Could you check a few things on this model? Use its own coordinates, in mm. A direction names the side the tool comes from. Coordinates: 2 decimals unless noted, no trailing zeros. One line per question, with ' | ' between items. Start each with the question number.
from build123d import *
from OCP.BRepFilletAPI import BRepFilletAPI_MakeChamfer

# Parameters (mm, degrees)
SKETCH1_W                       = 16.6
SKETCH1_H                       = 11.5
BOSS_EXTRUDE1_DEPTH             = 10
SKETCH2_W                       = 21
SKETCH2_H                       = 14.8
BOSS_EXTRUDE2_DEPTH             = 1.5
SKETCH3_W                       = 0.5
SKETCH3_H                       = 5
BOSS_EXTRUDE3_DEPTH             = 8
SKETCH4_W                       = 0.5
SKETCH4_H                       = 0.4
CUT_EXTRUDE1_DEPTH              = 22.623424798
BOSS_EXTRUDE4_REACH             = 19.241
SKETCH5_W                       = 0.75
SKETCH5_H                       = 2.5
BOSS_EXTRUDE4_DIRECTION_2_REACH = 19.241
BOSS_EXTRUDE5_DEPTH             = 2.8
BOSS_EXTRUDE5_DEPTH_BACK        = 2.8
CHAMFER1_SIZE                   = 1.8
CHAMFER1_SIZE2                  = 1.039230485
BOSS_EXTRUDE6_DEPTH             = 4.65
SKETCH9_W                       = 1.1
SKETCH9_H                       = 0.45
BOSS_EXTRUDE7_DEPTH             = 1.9
CHAMFER2_SIZE                   = 0.5
CHAMFER2_SIZE2                  = 0.288675135
SCALE2_SCALE                    = 0.7


with BuildPart() as part:
    # Sketch1 → Boss-Extrude1 (new body)
    with BuildSketch(Plane.XY):
        Rectangle(SKETCH1_W, SKETCH1_H)
    extrude(amount=BOSS_EXTRUDE1_DEPTH)

    # Sketch2 → Boss-Extrude2 (add)
    with BuildSketch(Plane.XY.offset(10)):
        Rectangle(SKETCH2_W, SKETCH2_H)
    extrude(amount=BOSS_EXTRUDE2_DEPTH)

    # Sketch3 → Boss-Extrude3 (add)
    with BuildSketch(Plane(origin=(0, 0, 0), x_dir=(-1, 0, 0), z_dir=(0, 0, -1))):
        with Locations((-6, 0)):
            Rectangle(SKETCH3_W, SKETCH3_H)
        Rectangle(SKETCH3_W, SKETCH3_H)
    extrude(amount=BOSS_EXTRUDE3_DEPTH)

    # Sketch4 → Cut-Extrude1 (cut, through all)
    with BuildSketch(Plane(origin=(6.25, 0, 0), x_dir=(0, 0, -1), z_dir=(1, 0, 0))):
        with Locations((2.25, 2.3)):
            Rectangle(SKETCH4_W, SKETCH4_H)
        with BuildLine():
            Line((0, 0.75), (0, -0.75))
            ThreePointArc((0, -0.75), (0.75, 0), (0, 0.75))
        make_face()
        Polygon((6.5, 2.5), (8, 1.449688693), (8, 2.5), align=None)
        with BuildLine():
            Line((5.432692308, 0.612598863), (6.3, 0))
            Line((6.3, 0), (5.432692308, -0.612598863))
            ThreePointArc((5.432692308, -0.612598863), (4.25, 0), (5.432692308, 0.612598863))
        make_face()
        Polygon((8, -2.5), (8, -1.449688693), (6.5, -2.5), align=None)
        with Locations((2.25, -2.3)):
            Rectangle(SKETCH4_W, SKETCH4_H)
    extrude(amount=-CUT_EXTRUDE1_DEPTH, mode=Mode.SUBTRACT)

    # Boss-Extrude4: up to this face of the body (flat: up to its plane)
    boss_extrude4_end = Plane(part.part.faces().sort_by_distance((0, 5.75, 5))[0])
    # Sketch5 → Boss-Extrude4 (add, up to the picked face)
    with BuildSketch(Plane(origin=(0, 0, 0), x_dir=(1, 0, 0), z_dir=(0, 1, 0)), mode=Mode.PRIVATE) as boss_extrude4_sk1:
        with Locations((-8.675, -1.25)):
            Rectangle(SKETCH5_W, SKETCH5_H)
    boss_extrude4_tool1 = split(extrude(boss_extrude4_sk1.sketch, amount=BOSS_EXTRUDE4_REACH, mode=Mode.PRIVATE), bisect_by=boss_extrude4_end, keep=Keep.BOTH, mode=Mode.PRIVATE)
    boss_extrude4 = boss_extrude4_tool1.solids().sort_by(Axis((-8.675, 0, 1.25), (0, 1, 0)))[0]
    add(boss_extrude4)

    # Boss-Extrude4 direction 2: up to this face of the body (flat: up to its plane)
    boss_extrude4_direction_2_end = Plane(part.part.faces().sort_by_distance((0, -5.75, 5))[0])
    # Sketch5 → Boss-Extrude4 direction 2 (add, up to the picked face)
    with BuildSketch(Plane(origin=(0, 0, 0), x_dir=(1, 0, 0), z_dir=(0, 1, 0)), mode=Mode.PRIVATE) as boss_extrude4_direction_2_sk1:
        with Locations((-8.675, -1.25)):
            Rectangle(SKETCH5_W, SKETCH5_H)
    boss_extrude4_direction_2_tool1 = split(extrude(boss_extrude4_direction_2_sk1.sketch, amount=-BOSS_EXTRUDE4_DIRECTION_2_REACH, mode=Mode.PRIVATE), bisect_by=boss_extrude4_direction_2_end, keep=Keep.BOTH, mode=Mode.PRIVATE)
    boss_extrude4_direction_2 = boss_extrude4_direction_2_tool1.solids().sort_by(Axis((-8.675, 0, 1.25), (0, -1, 0)))[0]
    add(boss_extrude4_direction_2)

    # Mirror1: Boss-Extrude4, Boss-Extrude4 direction 2 across plane
    add(boss_extrude4.mirror(Plane(origin=(0, 0, 0), x_dir=(0, 0, 1), z_dir=(1, 0, 0))))
    add(boss_extrude4_direction_2.mirror(Plane(origin=(0, 0, 0), x_dir=(0, 0, 1), z_dir=(1, 0, 0))))

    # Sketch6 → Boss-Extrude5 (add, two sides: drawn at the far end of the back side and taken through both)
    with BuildSketch(Plane(origin=(0, 0, 0), x_dir=(1, 0, 0), z_dir=(0, 1, 0)).offset(-BOSS_EXTRUDE5_DEPTH_BACK)):
        with BuildLine():
            Line((-9.05, -2.5), (-10.124907983, -5.653347952))
            ThreePointArc((-10.124907983, -5.653347952), (-10.231819447, -6.312838644), (-10.115557515, -6.970745323))
            Line((-10.115557515, -6.970745323), (-9.056614332, -9.938626949))
            Line((-9.056614332, -9.938626949), (-9.034716365, -10))
            Line((-9.034716365, -10), (-8.3, -10))
            Line((-8.3, -10), (-8.3, -9.827371619))
            Line((-8.3, -9.827371619), (-8.350231447, -9.686588817))
            Line((-8.350231447, -9.686588817), (-9.438479941, -6.636573707))
            ThreePointArc((-9.438479941, -6.636573707), (-9.496610907, -6.307620368), (-9.443155175, -5.977875022))
            Line((-9.443155175, -5.977875022), (-8.34011069, -2.741985882))
            Line((-8.34011069, -2.741985882), (-8.3, -2.624317241))
            Line((-8.3, -2.624317241), (-8.3, -2.5))
            Line((-8.3, -2.5), (-9.05, -2.5))
        make_face()
        with BuildLine():
            Line((8.3, -9.827371619), (8.350231447, -9.686588817))
            Line((8.350231447, -9.686588817), (9.438479941, -6.636573707))
            ThreePointArc((9.438479941, -6.636573707), (9.496610907, -6.307620368), (9.443155175, -5.977875022))
            Line((9.443155175, -5.977875022), (8.34011069, -2.741985882))
            Line((8.34011069, -2.741985882), (8.3, -2.624317241))
            Line((8.3, -2.624317241), (8.3, -2.5))
            Line((8.3, -2.5), (9.05, -2.5))
            Line((9.05, -2.5), (10.124907983, -5.653347952))
            ThreePointArc((10.124907983, -5.653347952), (10.231819447, -6.312838644), (10.115557515, -6.970745323))
            Line((10.115557515, -6.970745323), (9.056614332, -9.938626949))
            Line((9.056614332, -9.938626949), (9.034716365, -10))
            Line((9.034716365, -10), (8.3, -10))
            Line((8.3, -10), (8.3, -9.827371619))
        make_face()
    extrude(amount=BOSS_EXTRUDE5_DEPTH + BOSS_EXTRUDE5_DEPTH_BACK)

    # Chamfer1
    chamfer1_edges = [part.edges().sort_by_distance(p)[0] for p in [
        (10.5, 0, 11.5),
        (0, 7.4, 11.5),
        (-10.5, 0, 11.5),
        (0, -7.4, 11.5),
    ]]
    chamfer1_side = [part.faces().sort_by_distance(p)[0] for p in [
        (0, 0, 11.5),
    ]]
    chamfer(chamfer1_edges, length=CHAMFER1_SIZE, length2=CHAMFER1_SIZE2, reference=chamfer1_side[0])

    # Sketch7 → Boss-Extrude6 (add, symmetric)
    with BuildSketch(Plane(origin=(0, 0, 0), x_dir=(1, 0, 0), z_dir=(0, 1, 0))):
        with BuildLine():
            Line((-7.2, -11.5), (-3.398718251, -16.8))
            add(Edge.make_bspline(
                [(-3.398718251, -16.8), (0.927387699, -12.334784825), (7.2, -11.5)],
                knots=[0, 0, 0, 1, 1, 1], degree=2))
            Line((7.2, -11.5), (-7.2, -11.5))
        make_face()
    extrude(amount=BOSS_EXTRUDE6_DEPTH, both=True)

    # Sketch9 → Boss-Extrude7 (add)
    with BuildSketch(Plane(origin=(0, 0, 10), x_dir=(-1, 0, 0), z_dir=(0, 0, -1))):
        with Locations((-7.425, 5.975)):
            Rectangle(SKETCH9_W, SKETCH9_H)
        with Locations((-2.475, 5.975)):
            Rectangle(SKETCH9_W, SKETCH9_H)
        with Locations((2.475, 5.975)):
            Rectangle(SKETCH9_W, SKETCH9_H)
        with Locations((7.425, 5.975)):
            Rectangle(SKETCH9_W, SKETCH9_H)
        with Locations((7.425, -5.975)):
            Rectangle(SKETCH9_W, SKETCH9_H)
        with Locations((2.475, -5.975)):
            Rectangle(SKETCH9_W, SKETCH9_H)
        with Locations((-2.475, -5.975)):
            Rectangle(SKETCH9_W, SKETCH9_H)
        with Locations((-7.425, -5.975)):
            Rectangle(SKETCH9_W, SKETCH9_H)
    extrude(amount=BOSS_EXTRUDE7_DEPTH)

    # Chamfer2: one chamfer whose edges measure the first distance from different faces: ONE call of the kernel's chamfer builder (chamfer() names one face for all edges)
    chamfer2_edges_1 = [part.edges().sort_by_distance(p)[0] for p in [
        (7.425, 6.2, 8.1),
    ]]
    chamfer2_side_1 = [part.faces().sort_by_distance(p)[0] for p in [
        (7.425, 6.2, 9.05),
    ]]
    chamfer2_edges_2 = [part.edges().sort_by_distance(p)[0] for p in [
        (2.475, 6.2, 8.1),
    ]]
    chamfer2_side_2 = [part.faces().sort_by_distance(p)[0] for p in [
        (2.475, 6.2, 9.05),
    ]]
    chamfer2_edges_3 = [part.edges().sort_by_distance(p)[0] for p in [
        (-2.475, 6.2, 8.1),
    ]]
    chamfer2_side_3 = [part.faces().sort_by_distance(p)[0] for p in [
        (-2.475, 6.2, 9.05),
    ]]
    chamfer2_edges_4 = [part.edges().sort_by_distance(p)[0] for p in [
        (-7.425, 6.2, 8.1),
    ]]
    chamfer2_side_4 = [part.faces().sort_by_distance(p)[0] for p in [
        (-7.425, 6.2, 9.05),
    ]]
    chamfer2_edges_5 = [part.edges().sort_by_distance(p)[0] for p in [
        (-7.425, -6.2, 8.1),
    ]]
    chamfer2_side_5 = [part.faces().sort_by_distance(p)[0] for p in [
        (-7.425, -6.2, 9.05),
    ]]
    chamfer2_edges_6 = [part.edges().sort_by_distance(p)[0] for p in [
        (-2.475, -6.2, 8.1),
    ]]
    chamfer2_side_6 = [part.faces().sort_by_distance(p)[0] for p in [
        (-2.475, -6.2, 9.05),
    ]]
    chamfer2_edges_7 = [part.edges().sort_by_distance(p)[0] for p in [
        (2.475, -6.2, 8.1),
    ]]
    chamfer2_side_7 = [part.faces().sort_by_distance(p)[0] for p in [
        (2.475, -6.2, 9.05),
    ]]
    chamfer2_edges_8 = [part.edges().sort_by_distance(p)[0] for p in [
        (7.425, -6.2, 8.1),
    ]]
    chamfer2_side_8 = [part.faces().sort_by_distance(p)[0] for p in [
        (7.425, -6.2, 9.05),
    ]]
    chamfer2 = BRepFilletAPI_MakeChamfer(part.part.solid().wrapped)
    for e in chamfer2_edges_1:
        chamfer2.Add(CHAMFER2_SIZE, CHAMFER2_SIZE2, e.wrapped, chamfer2_side_1[0].wrapped)  # the first distance lies on this face
    for e in chamfer2_edges_2:
        chamfer2.Add(CHAMFER2_SIZE, CHAMFER2_SIZE2, e.wrapped, chamfer2_side_2[0].wrapped)  # the first distance lies on this face
    for e in chamfer2_edges_3:
        chamfer2.Add(CHAMFER2_SIZE, CHAMFER2_SIZE2, e.wrapped, chamfer2_side_3[0].wrapped)  # the first distance lies on this face
    for e in chamfer2_edges_4:
        chamfer2.Add(CHAMFER2_SIZE, CHAMFER2_SIZE2, e.wrapped, chamfer2_side_4[0].wrapped)  # the first distance lies on this face
    for e in chamfer2_edges_5:
        chamfer2.Add(CHAMFER2_SIZE, CHAMFER2_SIZE2, e.wrapped, chamfer2_side_5[0].wrapped)  # the first distance lies on this face
    for e in chamfer2_edges_6:
        chamfer2.Add(CHAMFER2_SIZE, CHAMFER2_SIZE2, e.wrapped, chamfer2_side_6[0].wrapped)  # the first distance lies on this face
    for e in chamfer2_edges_7:
        chamfer2.Add(CHAMFER2_SIZE, CHAMFER2_SIZE2, e.wrapped, chamfer2_side_7[0].wrapped)  # the first distance lies on this face
    for e in chamfer2_edges_8:
        chamfer2.Add(CHAMFER2_SIZE, CHAMFER2_SIZE2, e.wrapped, chamfer2_side_8[0].wrapped)  # the first distance lies on this face
    add(Compound.cast(chamfer2.Shape()), mode=Mode.REPLACE)


with BuildPart() as part_1:
    # Scale2: scaled about (-0.155191281, 0, 6.532138607)
    add(part.part.scale(SCALE2_SCALE).moved(Location((-0.046557384, 0, 1.959641582))))


solid = part_1.part
(1) On a 3-axis mill with a long thin cutter (end or side, diameter ignored), from which of +Z, -Z, +X, -X, +Y, -Y can I reach the whole of each face in a straight line? I mean faces 4 (the flat face through (6.75, -1.96, 6.3)), 5 (the flat face through (-7, 1.96, 6)), 6 (the flat face through (0, -5, 8.96)). Say none if no direction works.
(2) For P1, Ø1.5, axis at x = 2.5, z = 6, coming from the +Y side (3 decimals); P2, Ø1, axis at x = -0.5, y = -1, coming from the +Z side; P3, Ø3, axis at x = -3, y = 3, coming from the -Z side, each with a flat end and sliding along its axis, tell me the tip position at first contact or that it passes through.
(3) If I drill on line 1 along X through (y, z) = (1.5, 7.5); line 2 along X through (y, z) = (1, 7); line 3 along Z through (x, y) = (3.5, 3.75), over which ranges is the centre line in solid material (lowest first)? Write a range as from..to.
(4) We'd pull the mould along X, two halves only. Please class faces 1 (the flat face through (5.763, 0, 6)), 2 (the flat face through (-3.775, 0.046, 11.839)), 3 (the flat face through (6.68, -0.07, 9.64)): +X half, -X half, draft (parallel to the pull), parting line (faces both ways), or undercut.
Answers:
1) face 4: +X, -Y | face 5: -X, +Y | face 6: none
2) P1: y = 4.025 | P2: z = 12.45 | P3: z = 1.96
3) line 1: -6.89..-6.33, -5.86..5.76, 6.24..6.8 | line 2: -7.07..-6.51, -5.86..5.76, 6.42..6.98 | line 3: 1.96..10.01
4) face 1: undercut | face 2: -X half | face 3: +X half
